Build history of the part. All positions in model axes, mm. A direction names the side the tool comes from. Round coordinates to 2 decimals unless told otherwise and drop trailing zeros. Write each loop counter-clockwise with the first axis right and the second up, starting at its lowest first coordinate (ties: lowest second). Pieces come first, ordered by that corner, then holes. Notation, with made-up numbers: M 39.5,-26.5 L 94.5,-26.5 A17 cw 94.5,-0.5 Z; hole C 84.5,-1.5 d11. An arc over 180 degrees is marked long. Write item = value, one per line. Start each with the question number.
Q1. Band-saw the part on A-A on z = -29. Write the cut outline in (x, y), plus the area to 3 significant figures.
Q2. Band-saw the part on D-D on z = -17.5. Write the cut outline in (x, y).
Q3. Pull direction Z, two halves, no side cores. Call faces 6 (the cylindrical face through (3.29, 1.97, -5.38)), 7 (the flat face through (19.97, 10.02, -35.38)), 8 (the flat face through (3, 2, 0)): released by +Z, released by -Z, zero draft, split by the parting line, or undercut.
Q4. Band-saw the part on C-C on z = -5. Write the cut outline in (x, y) (3 decimals), plus the area to 3 significant figures.
Q5. Tool access for faces 1 (the flat face through (0, 2, -5)), 2 (the flat face through (27, 4, -25)), 3 (the flat face through (20, 4, -11)), 4 (the flat face through (13, 4, -25)), 5 (the flat face through (20, 0, -11)): list every direction of +Z, -Z, +X, -X, +Y, -Y with a clear straight run to the whole face (end or side of a thin tool).
Q6. Probe L1, parallel to X at y = 7.25, z = -29; L2, parallel to Y at x = 7.5, z = -7.5; L3, parallel to Y at x = 25, z = -33.5. List the from-to ranges inside material, lowest first.
Q7. Drop flat-ended pins along their axis: P1, Ø3, axis at x = 5, z = -5, coming from the -Y side; P2, Ø4.5, axis at y = 4.5, z = -25, coming from the +X side; P3, Ø8, axis at x = 20, z = -26.5, coming from the +Y side; P4, Ø3, axis at x = 13, z = -11, coming from the -Y side. Give the stop position or say it passes through.
Q8. Band-saw the part on B-B on x = 4.5. Write the cut outline in (y, z), plus the area to 3 significant figures.
```python
from build123d import *

# Parameters (mm, degrees)
SKETCH1_R                = 1.75
SKETCH1_W                = 14
SKETCH1_H                = 5
BOSS_EXTRUDE1_DEPTH      = 4
BOSS_EXTRUDE2_DEPTH      = 4
BOSS_EXTRUDE2_DEPTH_BACK = 12
SKETCH4_W                = 14
SKETCH4_H                = 4
SKETCH5_W                = 16
SKETCH5_H                = 3.464101615
CUT_EXTRUDE1_DEPTH       = 14
CUT_EXTRUDE2_DEPTH       = 14
FILLET1_R                = 5


with BuildPart() as part:
    # Sketch1 → Boss-Extrude1 (new body)
    # profile 1 of 2: a face of its own
    with BuildSketch(Plane(origin=(0, 0, 0), x_dir=(1, 0, 0), z_dir=(0, 1, 0))):
        with BuildLine():
            Line((40, 10), (27, 20))
            Line((27, 20), (13, 20))
            Line((13, 20), (0, 10))
            Line((0, 10), (0, 0))
            Line((0, 0), (5.717143143, 0))
            ThreePointArc((5.717143143, 0), (20, 6), (34.282856857, 0))
            Line((34.282856857, 0), (40, 0))
            Line((40, 0), (40, 10))
        make_face()
        with Locations(Location((5, 5, 0), (0, 0, 270))):
            Circle(SKETCH1_R, mode=Mode.SUBTRACT)
        with Locations(Location((35, 5, 0), (0, 0, 270))):
            Circle(SKETCH1_R, mode=Mode.SUBTRACT)
    # profile 2 of 2: a face of its own
    with BuildSketch(Plane(origin=(0, 0, 0), x_dir=(1, 0, 0), z_dir=(0, 1, 0))):
        with Locations((20, 22.5)):
            Rectangle(SKETCH1_W, SKETCH1_H)
    extrude(amount=BOSS_EXTRUDE1_DEPTH)

    # Sketch4 → Boss-Extrude2 (add, two sides: drawn at the far end of the back side and taken through both)
    with BuildSketch(Plane(origin=(0, 11.825317547, -20.482050808), x_dir=(1, 0, 0), z_dir=(0, -0.5000000000000041, 0.8660254037844364)).offset(-BOSS_EXTRUDE2_DEPTH_BACK)):
        with Locations((20, -9.035898385)):
            Rectangle(SKETCH4_W, SKETCH4_H)
    extrude(amount=BOSS_EXTRUDE2_DEPTH + BOSS_EXTRUDE2_DEPTH_BACK)

    # Sketch5 → Cut-Extrude1 (cut)
    with BuildSketch(Plane(origin=(0, 11.825317547, -20.482050808), x_dir=(1, 0, 0), z_dir=(0, -0.5000000000000041, 0.8660254037844364))):
        with Locations((21, -12.767949193)):
            Rectangle(SKETCH5_W, SKETCH5_H)
    extrude(amount=CUT_EXTRUDE1_DEPTH, mode=Mode.SUBTRACT)

    # Sketch6 → Cut-Extrude2 (cut)
    with BuildSketch(Plane(origin=(0, -6.09326674, -3.517949192), x_dir=(1, 0, 0), z_dir=(0, 0.8660254037844364, 0.5000000000000041))):
        with BuildLine():
            Line((18, 24.407537572), (18, 30.650635095))
            ThreePointArc((18, 30.650635095), (20, 32.650635095), (22, 30.650635095))
            Line((22, 30.650635095), (22, 24.407537572))
            ThreePointArc((22, 24.407537572), (20, 22.407537572), (18, 24.407537572))
        make_face()
    extrude(amount=-CUT_EXTRUDE2_DEPTH, mode=Mode.SUBTRACT)

    # Fillet1
    fillet1_edges = [part.edges().sort_by_distance(p)[0] for p in [
        (13, 10, -35.392304845),
        (27, 10, -35.392304845),
    ]]
    fillet(fillet1_edges, radius=FILLET1_R)


solid = part.part
```
Conclusion:
q1.outline = M 13,4 L 18,4 L 18,8.62 L 13,8.62 Z; M 22,4 L 27,4 L 27,8.62 L 22,8.62 Z
q1.area = 46.2 mm^2
q2.outline = M 9.75,0 L 30.25,0 L 30.25,4 L 9.75,4 Z
q3.face_6 = undercut
q3.face_7 = released by -Z
q3.face_8 = released by +Z
q4.outline = M 0,0 L 3.25,0 L 3.25,4 L 0,4 Z; M 6.75,0 L 13.755,0 L 13.755,4 L 6.75,4 Z; M 26.245,0 L 33.25,0 L 33.25,4 L 26.245,4 Z; M 36.75,0 L 40,0 L 40,4 L 36.75,4 Z
q4.area = 82.0 mm^2
q5.face_1 = +Z, -Z, -X, +Y, -Y
q5.face_2 = -Z, +X, +Y, -Y
q5.face_3 = +Z, +X, -X, +Y
q5.face_4 = -Z, -X, +Y, -Y
q5.face_5 = +Z, -Z, +X, -X, -Y
q6.L1 = 13 to 18, 22 to 27
q6.L2 = 0 to 4
q6.L3 = 6.6 to 11.22
q7.P1 = through
q7.P2 = 27
q7.P3 = 9.18
q7.P4 = 0
q8.outline = M 0,-13.46 L 4,-13.46 L 4,-6.68 L 0,-6.68 Z; M 0,-3.32 L 4,-3.32 L 4,0 L 0,0 Z
q8.area = 40.4 mm^2
